```python
from build123d import *

# Parameters (mm, degrees)
SKETCH1_R           = 16.5
BOSS_EXTRUDE1_DEPTH = 4.4
BOSS_EXTRUDE2_DEPTH = 5.3
SKETCH3_R           = 3.6
CUT_EXTRUDE1_DEPTH  = 4.4
CUT_EXTRUDE2_DEPTH  = 4.4
SKETCH5_R           = 1.2
CUT_EXTRUDE3_DEPTH  = 319.076390196
SKETCH6_R           = 2.3
CUT_EXTRUDE4_DEPTH  = 3


with BuildPart() as part:
    # Sketch1 → Boss-Extrude1 (new body)
    with BuildSketch(Plane(origin=(204.9, 0, 0), x_dir=(0, 0, -1), z_dir=(1, 0, 0))):
        with Locations((-301, 0)):
            Circle(SKETCH1_R)
    extrude(amount=BOSS_EXTRUDE1_DEPTH)

    # Sketch2 → Boss-Extrude2 (add)
    with BuildSketch(Plane(origin=(209.3, 0, 0), x_dir=(0, 0, -1), z_dir=(1, 0, 0))):
        Polygon((-306.532, 1.019), (-307.966, 1.068), (-308.758, 1.491), (-309.431, 2.148), (-309.083, 3.218), (-308.153, 3.354), (-307.264, 3.23), (-306.074, 2.427), (-304.876, 4.076), (-306.008, 4.959), (-306.4, 5.766), (-306.558, 6.693), (-305.648, 7.354), (-304.815, 6.918), (-304.169, 6.295), (-303.679, 4.946), (-301.74, 5.576), (-302.137, 6.955), (-301.98, 7.839), (-301.563, 8.682), (-300.437, 8.682), (-300.02, 7.839), (-299.863, 6.955), (-300.26, 5.576), (-298.321, 4.946), (-297.831, 6.295), (-297.185, 6.918), (-296.352, 7.354), (-295.442, 6.693), (-295.6, 5.766), (-295.992, 4.959), (-297.124, 4.076), (-295.926, 2.427), (-294.736, 3.23), (-293.847, 3.354), (-292.917, 3.218), (-292.569, 2.148), (-293.242, 1.491), (-294.034, 1.068), (-295.468, 1.019), (-295.468, -1.019), (-294.034, -1.068), (-293.242, -1.491), (-292.569, -2.148), (-292.917, -3.218), (-293.847, -3.354), (-294.736, -3.23), (-295.926, -2.427), (-297.124, -4.076), (-295.992, -4.959), (-295.6, -5.766), (-295.442, -6.693), (-296.352, -7.354), (-297.185, -6.918), (-297.831, -6.295), (-298.321, -4.946), (-300.26, -5.576), (-299.863, -6.955), (-300.02, -7.839), (-300.437, -8.682), (-301.563, -8.682), (-301.98, -7.839), (-302.137, -6.955), (-301.74, -5.576), (-303.679, -4.946), (-304.169, -6.295), (-304.815, -6.918), (-305.648, -7.354), (-306.558, -6.693), (-306.4, -5.766), (-306.008, -4.959), (-304.876, -4.076), (-306.074, -2.427), (-307.264, -3.23), (-308.153, -3.354), (-309.083, -3.218), (-309.431, -2.148), (-308.758, -1.491), (-307.966, -1.068), (-306.532, -1.019), align=None)
    extrude(amount=BOSS_EXTRUDE2_DEPTH)

    # Sketch3 → Cut-Extrude1 (cut)
    with BuildSketch(Plane(origin=(204.9, 0, 0), x_dir=(0, 0, -1), z_dir=(1, 0, 0))):
        with Locations((-301, 0)):
            Circle(SKETCH3_R)
    extrude(amount=CUT_EXTRUDE1_DEPTH, mode=Mode.SUBTRACT)

    # Sketch4 → Cut-Extrude2 (cut)
    with BuildSketch(Plane(origin=(204.9, 0, 0), x_dir=(0, 0, -1), z_dir=(1, 0, 0))):
        Polygon((-285.15, -1.95), (-301, -2.8), (-316.85, -1.95), (-316.85, 1.95), (-301, 2.8), (-285.15, 1.95), align=None)
    extrude(amount=CUT_EXTRUDE2_DEPTH, mode=Mode.SUBTRACT)

    # Sketch5 → Cut-Extrude3 (cut, through all)
    with BuildSketch(Plane(origin=(204.9, 0, 0), x_dir=(0, 0, -1), z_dir=(1, 0, 0))):
        with Locations((-301, 0)):
            Circle(SKETCH5_R)
    extrude(amount=CUT_EXTRUDE3_DEPTH, mode=Mode.SUBTRACT)

    # Sketch6 → Cut-Extrude4 (cut)
    with BuildSketch(Plane(origin=(214.6, 0, 0), x_dir=(0, 0, -1), z_dir=(1, 0, 0))):
        with Locations((-301, 0)):
            Circle(SKETCH6_R)
    extrude(amount=-CUT_EXTRUDE4_DEPTH, mode=Mode.SUBTRACT)


solid = part.part
```
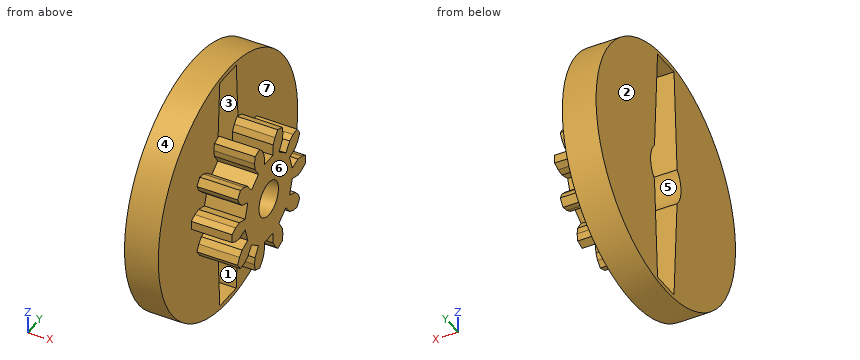
Geometry check sheet. Reference: the model listing, model coordinates, mm. Face numbers are marked on the shaded views. A direction names the side the tool comes from. Coordinates: 2 decimals unless noted, no trailing zeros. Write each loop counter-clockwise with the first axis right and the second up, starting at its lowest first coordinate (ties: lowest second). Pieces come first, ordered by that corner, then holes. Notation, with made-up numbers: M -21.5,-0.5 L 31.5,-0.5 A12 ccw 31.5,10.5 Z; hole C 77.25,1.5 d1. An arc over 180 degrees is marked long. Answer as a JSON object with one key per item and string values.
1. Section check D-D, the plane y = -13.5. Enter the section's corners in (x, z).
Answers below:
{"outline": "M 204.9,291.51 L 209.3,291.51 L 209.3,310.49 L 204.9,310.49 Z"}
2. Draft check along Z on the marked faces 1, 2, 3 and 4. Enter one of: released by +Z, released by -Z, zero draft, split by the parting line, or undercut.
Answers below:
{"face 1": "undercut", "face 2": "zero draft", "face 3": "undercut", "face 4": "split by the parting line"}
3. Section check A-A, the plane y = 0. Enter the section's corners in (x, z).
Answers below:
{"outline": "M 204.9,284.5 L 209.3,284.5 L 209.3,285.15 L 204.9,285.15 Z; M 204.9,316.85 L 209.3,316.85 L 209.3,317.5 L 204.9,317.5 Z; M 209.3,295.47 L 214.6,295.47 L 214.6,298.7 L 211.6,298.7 L 211.6,299.8 L 209.3,299.8 Z; M 209.3,302.2 L 211.6,302.2 L 211.6,303.3 L 214.6,303.3 L 214.6,306.53 L 209.3,306.53 Z"}
4. Go/stop test with flat-tipped pins: pin 1 Ø5 at (x, y) = (213.5, -7) entering from -Z; pin 2 Ø1 at (x, z) = (213.5, 295.5) entering from -Y; pin 3 Ø0.9 at (x, z) = (211.5, 301) entering from -Y; pin 4 Ø2 at (y, z) = (0, 301) entering from -X. Record where each tip stops, or that it passes through.
Answers below:
{"pin 1": "stops at z = 295.44", "pin 2": "stops at y = -7.1", "pin 3": "stops at y = -8.68", "pin 4": "passes through"}
5. Section check B-B, the plane z = 301. Enter the section's corners in (x, y), plus the area to 3 significant figures.
Answers below:
{"outline": "M 204.9,-16.5 L 209.3,-16.5 L 209.3,-8.68 L 214.6,-8.68 L 214.6,-2.3 L 211.6,-2.3 L 211.6,-1.2 L 209.3,-1.2 L 209.3,-3.6 L 204.9,-3.6 Z; M 204.9,3.6 L 209.3,3.6 L 209.3,1.2 L 211.6,1.2 L 211.6,2.3 L 214.6,2.3 L 214.6,8.68 L 209.3,8.68 L 209.3,16.5 L 204.9,16.5 Z", "area": "186 mm²"}
6. Tool access check on the marked faces 5, 6 and 7. Record the directions out of +Z, -Z, +X, -X, +Y, -Y that give a thin tool (end or side, any length) a straight path to the whole face; none if there is none.
Answers below:
{"face 5": "-X", "face 6": "+Z, -Z, +X, +Y, -Y", "face 7": "+X"}
7. Scan lines: L1, parallel to Y at x = 210.6, z = 301; L2, parallel to Z at x = 211.1, y = 0; L3, parallel to Z at x = 206.75, y = 0.5. Record each from-to range of solid material in increasing order.
Answers below:
{"L1": "y = -8.68 to -1.2, 1.2 to 8.68", "L2": "z = 295.47 to 299.8, 302.2 to 306.53", "L3": "z = 284.51 to 285.15, 316.85 to 317.49"}
8. Section check C-C, the plane x = 207.5. Enter the section's corners in (y, z), plus the area to 3 significant figures.
Answers below:
{"outline": "C 0,301 d33; hole M -2.67,298.59 L -1.95,285.15 L 1.95,285.15 L 2.67,298.59 A3.6 ccw 2.67,303.41 L 1.95,316.85 L -1.95,316.85 L -2.67,303.41 A3.6 ccw Z", "area": "699 mm²"}
